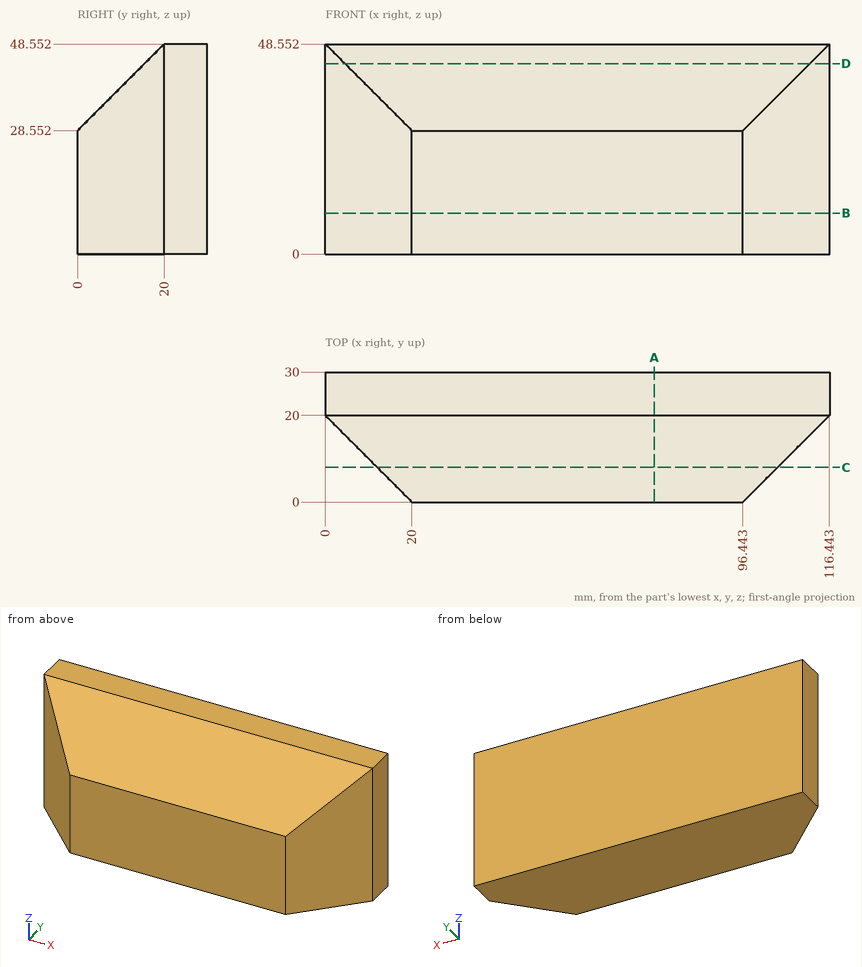
Verification items for this drawing (mm, ordinates from the low corner). Coordinates: 2 decimals unless noted, no trailing zeros. Write each loop counter-clockwise with the first axis right and the second up, starting at its lowest first coordinate (ties: lowest second). Pieces come first, ordered by that corner, then holes. Notation, with made-up numbers: M 5,-5.5 L 51,-5.5 A12 cw 51,4.5 Z; hole C -2,78.5 d9. An arc over 180 degrees is marked long. One line per item, written item: value. Start each with the question number.
(1) Depth check by flat-ended pin: pin 1 (12 mm diameter, centred on y = 5, z = 28, fed in from +X); pin 2 (1.5 mm diameter, centred on x = 61.5, y = 3.5, fed in from +Z); pin 3 (3 mm diameter, centred on y = 10.5, z = 15, fed in from -X). Enter the tip coordinate at first touch or a pass-through.
(2) Scan lines: line 1 along X through (y, z) = (16.5, 4); line 2 along Z through (x, y) = (29, 3); line 3 along Z through (x, y) = (101, 6.5). Record each from-to range of solid material in increasing order. Write a range as [from, to].
(3) Sectioned sample at C-C, the plane y = 8. Enter the section's corners in (x, z), and give its area (3 significant figures).
(4) Sectioned sample at D-D, the plane z = 44. Enter the section's corners in (x, y), and give its area (3 significant figures).
(5) Sectioned sample at B-B, the plane z = 9.5. Enter the section's corners in (x, y).
(6) Sectioned sample at A-A, the plane x = 76. Enter the section's corners in (y, z), and give its area (3 significant figures).
Filled sheet:
1. pin 1: x = 107.44
1. pin 2: z = 32.8
1. pin 3: x = 8
2. line 1: [3.5, 112.94]
2. line 2: [0, 31.55]
2. line 3: [0, 35.05]
3. outline: M 12,0 L 104.44,0 L 104.44,36.55 L 12,36.55 Z
3. area: 3,380 mm²
4. outline: M 0,20 L 4.55,15.45 L 111.89,15.45 L 116.44,20 L 116.44,30 L 0,30 Z
4. area: 1,670 mm²
5. outline: M 0,20 L 20,0 L 96.44,0 L 116.44,20 L 116.44,30 L 0,30 Z
6. outline: M 0,0 L 30,0 L 30,48.55 L 20,48.55 L 0,28.55 Z
6. area: 1,260 mm²
